Autodesk Inventor part; units mm, degrees
ref_plane "YZ Plane" through (0, 0, 0) normal (1, 0, 0) x (0, 1, 0)
ref_plane "XZ Plane" through (0, 0, 0) normal (0, 1, 0) x (-1, 0, 0)
ref_plane "XY Plane" through (0, 0, 0) normal (0, 0, 1) x (1, 0, 0)
sketch "Sketch1" plane through (0, 0, 0) normal (0, 0, 1) x (1, 0, 0)
  line L0 (0, 0) -> (88.9, 0)
  line L1 (88.9, 0) -> (88.9, 63.5)
  line L2 (88.9, 63.5) -> (0, 63.5)
  line L3 (0, 63.5) -> (0, 0)
  dimension "d0" = 88.9
  dimension "d1" = 63.5
extrude "Extrusion1" add sketch "Sketch1" along normal blind 3.175
sketch "Sketch2" plane through (0, 0, 3.175) normal (0, 0, 1) x (1, 0, 0)
  line L0 (0, 0) -> (0, 63.5)
  line L1 (88.9, 0) -> (0, 0)
  circle A0 centre (19.05, 25.4) radius 9.525
  dimension "d4" = 19.05
  dimension "d5" = 19.05
  dimension "d6" = 25.4
extrude "Extrusion2" cut sketch "Sketch2" against normal through all
properties part number "Plate_VerticalRollerMount_Bottom"
Can you work these out from the model? Positions are in its coordinate system, mm. Round coordinates to 2 decimals unless told otherwise and drop trailing zeros. Loops run counter-clockwise (first coordinate to the right, second up) from the corner with the lowest first, then second, coordinate; pieces in that order, holes last. Notation, with made-up numbers: M -3,86 L 37,86 A21 cw 37,90 Z; hole C 0.25,16 d1. An arc over 180 degrees is marked long. Answer as a JSON object with one key per item and string values. Group by question number.
Q1. Imagine slicing it at C-C, the plane z = 1. Please give me the cut outline in (x, y) (3 decimals).
Q2. Imagine slicing it at A-A, the plane y = 25.4. Please give me the cut outline in (x, z) (3 decimals), then the cut area to 3 significant figures.
Q3. Please list where these lines run through material, in increasing order: L1, parallel to Y at x = 19.05, z = 0.75 (3 decimals); L2, parallel to X at y = 29, z = 1.9; L3, parallel to X at y = 18.5, z = 1.1.
Q4. Imagine slicing it at B-B, the plane x = 19.05. Please give me the cut outline in (y, z) (3 decimals).
Q5. We'd pull the mould along X, two halves only. Please class faces 1 (the flat face through (0, 32, 2)), 2 (the flat face through (44, 32, 3.175)), 3 (the cylindrical face through (17, 16.1, 1.6)): +X half, -X half, draft (parallel to the pull), parting line (faces both ways), or undercut.
Findings:
{
 "1": {"outline": "M 0,0 L 88.9,0 L 88.9,63.5 L 0,63.5 Z; hole C 19.05,25.4 d19.05"},
 "2": {"outline": "M 0,0 L 9.525,0 L 9.525,3.175 L 0,3.175 Z; M 28.575,0 L 88.9,0 L 88.9,3.175 L 28.575,3.175 Z", "area": "222 mm2"},
 "3": {"L1": "y = 0 to 15.875, 34.925 to 63.5", "L2": "x = 0 to 10.23, 27.87 to 88.9", "L3": "x = 0 to 12.48, 25.62 to 88.9"},
 "4": {"outline": "M 0,0 L 15.875,0 L 15.875,3.175 L 0,3.175 Z; M 34.925,0 L 63.5,0 L 63.5,3.175 L 34.925,3.175 Z"},
 "5": {"face 1": "-X half", "face 2": "draft", "face 3": "undercut"}
}
